The model under review builds one solid part; all positions refer to its coordinate system, in mm. A direction names the side the tool comes from. Coordinates: 2 decimals unless noted, no trailing zeros. Order: outer loops, then holes, each group sorted by start corner. A loop starts at its lowest first (then second) coordinate and runs counter-clockwise, first axis right, second up.
```python
from build123d import *

# Parameters (mm, degrees)
SKETCH2_R           = 12.5
BOSS_EXTRUDE1_DEPTH = 120
SKETCH3_R           = 5
BOSS_EXTRUDE2_DEPTH = 10


with BuildPart() as part:
    # Sketch2 → Boss-Extrude1 (new body)
    with BuildSketch(Plane.XY):
        Circle(SKETCH2_R)
    extrude(amount=-BOSS_EXTRUDE1_DEPTH)

    # Sketch3 → Boss-Extrude2 (add)
    with BuildSketch(Plane.XY):
        Circle(SKETCH3_R)
    boss_extrude2 = extrude(amount=BOSS_EXTRUDE2_DEPTH)

    # Mirror1: Boss-Extrude2 across plane
    add(boss_extrude2.mirror(Plane.XY.offset(-60)))


solid = part.part
```
(1) We need section A-A, the plane x = 0. Write out the cut boundary in (y, z), and give its area (3 significant figures).
A:
outline: (-12.5, -120) - (-5, -120) - (-5, -130) - (5, -130) - (5, -120) - (12.5, -120) - (12.5, 0) - (5, 0) - (5, 10) - (-5, 10) - (-5, 0) - (-12.5, 0) - close
area: 3,200 mm2
(2) We need section D-D, the plane y = -7.5. Write out the cut boundary in (x, z).
A:
outline: (-10, -120) - (10, -120) - (10, 0) - (-10, 0) - close
(3) We need section C-C, the plane z = -80. Write out the cut boundary in (x, y), and give its area (3 significant figures).
A:
outline: circle Ø25 at (0, 0)
area: 491 mm2
(4) Machinability: for faces 1 (the face through (-1.08, -4.88, 4.93)), 2 (the face through (-1.08, -4.88, -124.93)), 3 (the face through (0, 0, 10)), which of the approach directions +Z, -Z, +X, -X, +Y, -Y give a long, thin tool a straight path to every point of the face, cutting with its end or side? Answer none if there is none.
A:
face 1: +Z
face 2: -Z
face 3: +Z, +X, -X, +Y, -Y
(5) Wall thickness on probe 1 along Z at (x, y) = (-8.25, -2); probe 2 along Y at (x, z) = (-0.5, -45); probe 3 along Y at (x, z) = (1.25, -82): over which ranges is each line inside the solid? List them lowest first.
A:
probe 1: z = -120 to 0
probe 2: y = -12.49 to 12.49
probe 3: y = -12.44 to 12.44
(6) For pin 1 Ø4 at (y, z) = (-8.5, -46) entering from -X; pin 2 Ø1.5 at (y, z) = (-6.5, -99.5) entering from -X; pin 3 Ø4 at (x, z) = (-5, -39.5) entering from -Y; pin 4 Ø12 at (x, y) = (6, 9) entering from +Z, all flat-tipped, find the tip position at first contact; note any pin that passes through.
A:
pin 1: stops at x = -10.68
pin 2: stops at x = -11.1
pin 3: stops at y = -12.13
pin 4: stops at z = 10
